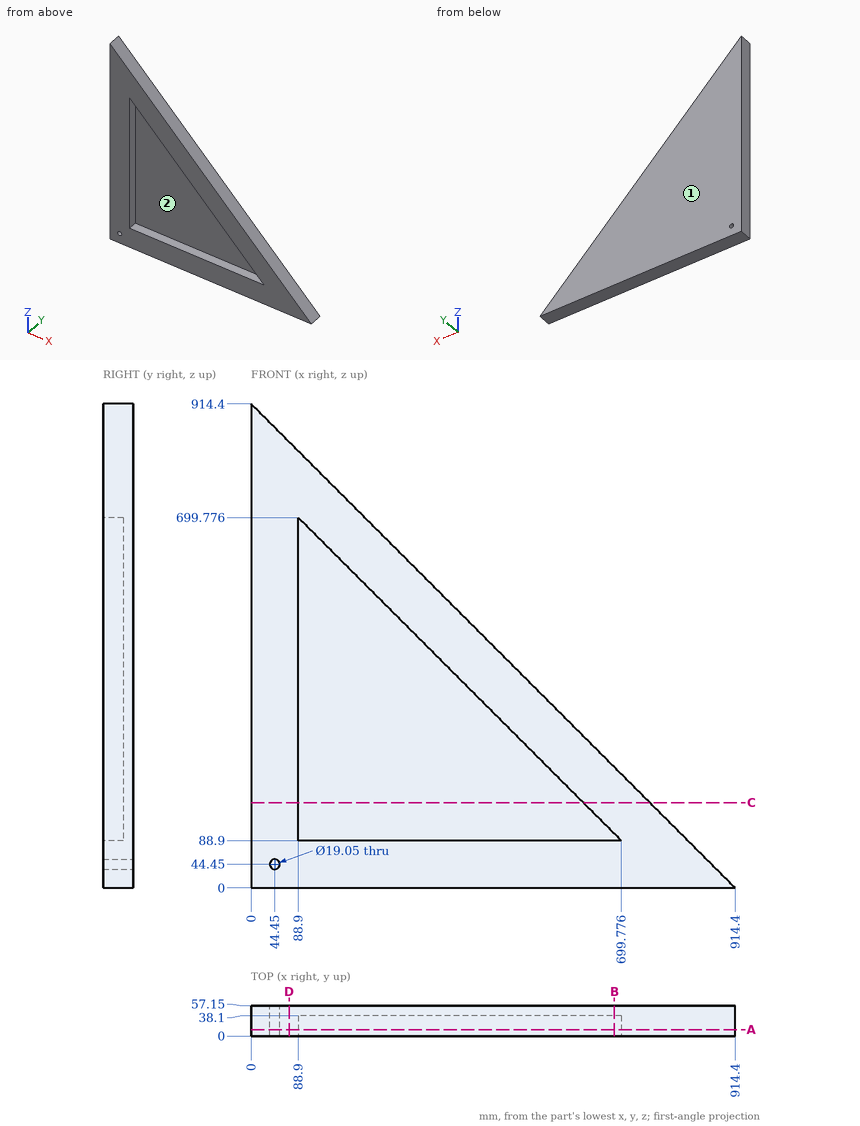
Geometry: see drawing. Coordinates: mm, zero at the bounding-box minimum. Round coordinates to 2 decimals unless told otherwise and drop trailing zeros. Write each loop counter-clockwise with the first axis right and the second up, starting at its lowest first coordinate (ties: lowest second). Pieces come first, ordered by that corner, then holes.
1) Ray query, L1, parallel to Y at x = 441, z = 208; L2, parallel to X at y = 33, z = 401.5 (1 decimal); L3, parallel to X at y = 22, z = 136 (1 decimal). Return the intervals inside material, ascending.
2) Cut plane B-B (x = 686.5). Return the cut outline in (y, z).
3) Cut plane A-A (y = 12). Count the separate pieces of the cut face and the enclosed holes in it, then the cut area to 3 significant figures.
4) Cut plane C-C (z = 161). Return the cut outline in (x, y).
5) Contact query for flat-ended pins moving along their axis: P1, Ø1, axis at x = 243.5, z = 143.5, coming from the -Y side; P2, Ø12, axis at x = 464, y = 6, coming from the -Z side; P3, Ø6, axis at y = 18, z = 783.5, coming from the +X side; P4, Ø11.5, axis at y = 17, z = 390, coming from the +X side. Output: stop coordinate, or through.
6) Cut plane D-D (x = 71.5). Return the cut outline in (y, z), then the cut area to 3 significant figures.
7) Draft query along X for the marked faces 1 and 2. Return one class per face: pulls with the +X half, pulls with the -X half, needs draft (parallel to the pull), parting line crosses it, or undercut.
Geometry says:
1. L1: y = 38.1 to 57.15
1. L2: x = 0 to 88.9, 387.2 to 512.9
1. L3: x = 0 to 88.9, 652.7 to 778.4
2. outline: (0, 0) - (57.15, 0) - (57.15, 227.9) - (0, 227.9) - (0, 102.18) - (38.1, 102.18) - (38.1, 88.9) - (0, 88.9) - close
3. separate pieces: 1
3. enclosed holes: 2
3. area: 231,000 mm2
4. outline: (0, 0) - (88.9, 0) - (88.9, 38.1) - (627.68, 38.1) - (627.68, 0) - (753.4, 0) - (753.4, 57.15) - (0, 57.15) - close
5. P1: stops at y = 38.1
5. P2: stops at z = 0
5. P3: stops at x = 133.9
5. P4: stops at x = 530.15
6. outline: (0, 0) - (57.15, 0) - (57.15, 842.9) - (0, 842.9) - close
6. area: 48,200 mm2
7. face 1: needs draft
7. face 2: undercut
